Verification items for the finished model (mm, model axes). Face numbers are marked on the shaded views. Give positions to 0.01 mm unless a question says otherwise; leave off trailing zeros. Loops run counter-clockwise (first coordinate to the right, second up) from the corner with the lowest first, then second, coordinate; pieces in that order, holes last. Notation, with made-up numbers: M 12.25,31.25 L 33.25,31.25 A33 cw 33.25,67.25 Z; hole C 12,37 d1. An arc over 180 degrees is marked long. Use a Markdown table: item, result.
from build123d import *

# Parameters (mm, degrees)
F0_R     = 25.4
F1_DEPTH = 50.8
F2_SIZE  = 5.08
F3_SIZE  = 5.08
F4_R     = 12.7
F5_DEPTH = 50.8


with BuildPart() as f1:
    # F0 (on Front) → F1 (new body)
    with BuildSketch(Plane.XZ):
        Circle(F0_R)
    extrude(amount=F1_DEPTH)

    # F2
    f2_edges = [f1.edges().sort_by_distance(p)[0] for p in [
        (-25.4, -50.8, 0),
    ]]
    chamfer(f2_edges, length=F2_SIZE)

    # F3
    f3_edges = [f1.edges().sort_by_distance(p)[0] for p in [
        (-25.4, 0, 0),
    ]]
    chamfer(f3_edges, length=F3_SIZE)

    # F4 (on Front) → F5 (cut)
    with BuildSketch(Plane.XZ):
        Circle(F4_R)
    extrude(amount=F5_DEPTH, mode=Mode.SUBTRACT)


solid = f1.part
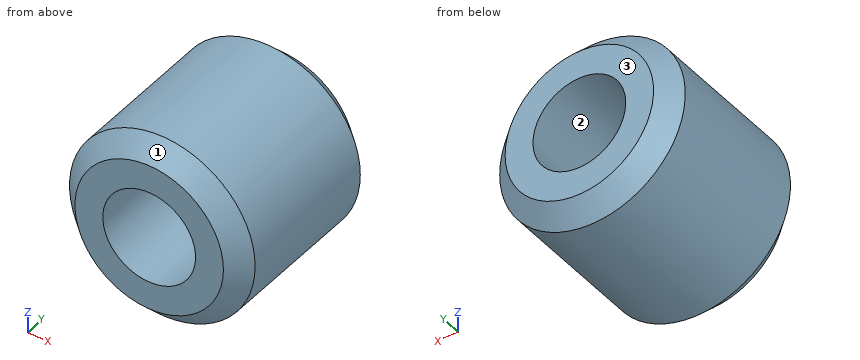
(1) Cross-section at B-B on z = 0. Record the cut outline in (x, y), then the cut area to 3 significant figures.
Results below:
| item | result |
|---|---|
| outline | M -25.4,-45.72 L -20.32,-50.8 L -12.7,-50.8 L -12.7,0 L -20.32,0 L -25.4,-5.08 Z; M 12.7,-50.8 L 20.32,-50.8 L 25.4,-45.72 L 25.4,-5.08 L 20.32,0 L 12.7,0 Z |
| area | 1,240 mm^2 |
(2) Cross-section at A-A on x = 0. Record the cut outline in (y, z), then the cut area to 3 significant figures.
Results below:
| item | result |
|---|---|
| outline | M -50.8,-20.32 L -45.72,-25.4 L -5.08,-25.4 L 0,-20.32 L 0,-12.7 L -50.8,-12.7 Z; M -50.8,12.7 L 0,12.7 L 0,20.32 L -5.08,25.4 L -45.72,25.4 L -50.8,20.32 Z |
| area | 1,240 mm^2 |
(3) Cross-section at C-C on y = -47. Record the cut outline in (x, z).
Results below:
| item | result |
|---|---|
| outline | C 0,0 d48.24; hole C 0,0 d25.4 |
(4) Draft check along X on the marked faces 1, 2 and 3. Enter one of: +X half, -X half, draft (parallel to the pull), parting line (faces both ways), or undercut.
Results below:
| item | result |
|---|---|
| face 1 | parting line |
| face 2 | undercut |
| face 3 | draft |
(5) Material ranges on line 1 (Z direction, x = 0, y = -27); line 2 (Z direction, x = -7, y = -15.5); line 3 (X direction, y = -37, z = 8.5), recorded low to high.
Results below:
| item | result |
|---|---|
| line 1 | -25.4 to -12.7, 12.7 to 25.4 |
| line 2 | -24.42 to -10.6, 10.6 to 24.42 |
| line 3 | -23.94 to -9.44, 9.44 to 23.94 |
(6) Gauge pin test, flat ends, axial feed: P1, Ø2, axis at y = -43.5, z = -5, coming from the +X side; P2, Ø12, axis at x = -13, y = -12.5, coming from the -Z side; P3, Ø5, axis at x = 12.5, y = -25, coming from the -Z side. Record the tip position at first contact, or that the pin passes through.
Results below:
| item | result |
|---|---|
| P1 | x = 25.08 |
| P2 | z = -24.42 |
| P3 | z = -23.35 |
